from build123d import *

# Parameters (mm, degrees)
F0_W      = 70
F0_H      = 100
F1_DEPTH  = 19
F3_DEPTH  = 3
F4_R      = 16
F5_DEPTH  = 3
F7_DEPTH  = 3
F8_R      = 2
F9_DEPTH  = 3
F10_R     = 2
F11_DEPTH = 3


with BuildPart() as f1:
    # F0 (on Front) → F1 (new body)
    with BuildSketch(Plane.XZ):
        with Locations((35, -50)):
            Rectangle(F0_W, F0_H)
    extrude(amount=F1_DEPTH)

    # F2 (on face) → F3 (join)
    with BuildSketch(Plane.XZ.offset(19)):
        with BuildLine():
            Line((57, -8), (12, -8))
            Line((12, -8), (8, -11.356399))
            Line((8, -11.356399), (8, -86.344417))
            Line((8, -86.344417), (13.655583, -92))
            Line((13.655583, -92), (59, -92))
            ThreePointArc((59, -92), (61.162278, -90.576506), (62, -88.127017))
            Line((62, -88.127017), (62, -13))
            ThreePointArc((62, -13), (60.535534, -9.464466), (57, -8))
        make_face()
    extrude(amount=F3_DEPTH)

    # F4 (on face) → F5 (cut)
    with BuildSketch(Plane.XZ.offset(22)):
        with Locations((35, -30)):
            Circle(F4_R)
    extrude(amount=-F5_DEPTH, mode=Mode.SUBTRACT)

    # F6 (on face) → F7 (cut)
    with BuildSketch(Plane.XZ.offset(22)):
        with BuildLine():
            Line((47.590841, -64.431946), (29.590728, -64.431946))
            ThreePointArc((29.590728, -64.431946), (25.361132, -66.176302), (23.590841, -70.395109))
            Line((23.590841, -70.395109), (23.541725, -78.395109))
            ThreePointArc((23.541725, -78.395109), (25.285967, -82.661543), (29.541612, -84.431946))
            Line((29.541612, -84.431946), (47.590841, -84.431946))
            ThreePointArc((47.590841, -84.431946), (51.833482, -82.674587), (53.590841, -78.431946))
            Line((53.590841, -78.431946), (53.590841, -70.431946))
            ThreePointArc((53.590841, -70.431946), (51.833482, -66.189306), (47.590841, -64.431946))
        make_face()
    extrude(amount=-F7_DEPTH, mode=Mode.SUBTRACT)

    # F8 (on face) → F9 (cut)
    with BuildSketch(Plane.XZ.offset(22)):
        with Locations((10.5, -31.813467)):
            Circle(F8_R)
        with Locations((18.186533, -39.5)):
            Circle(F8_R)
        with BuildLine():
            ThreePointArc((19, -50), (21, -52), (23, -50))
            ThreePointArc((23, -50), (21, -48), (19, -50))
        make_face()
        with Locations((18.186533, -60.5)):
            Circle(F8_R)
        with Locations((10.5, -68.186533)):
            Circle(F8_R)
    extrude(amount=-F9_DEPTH, mode=Mode.SUBTRACT)

    # F10 (on face) → F11 (cut)
    with BuildSketch(Plane.XZ.offset(22)):
        with Locations((56, -40)):
            Circle(F10_R)
        with Locations((55.891707, -50)):
            Circle(F10_R)
        with Locations((56, -60)):
            Circle(F10_R)
    extrude(amount=-F11_DEPTH, mode=Mode.SUBTRACT)


solid = f1.part
Work out the finished part from the listing and answer in its coordinate system (mm). A direction names the side the tool comes from. Round coordinates to 2 decimals unless told otherwise and drop trailing zeros. Order: outer loops, then holes, each group sorted by start corner. A loop starts at its lowest first (then second) coordinate and runs counter-clockwise, first axis right, second up. Notation, with made-up numbers: M 27.25,26.25 L 60.25,26.25 A20 ccw 60.25,56.25 Z; hole C 15.5,-32.5 d11. An arc over 180 degrees is marked long. Put each result on its own line as item: value. Start each with the question number.
Q1. Section C-C, the plane y = -20 is taken. Give the number of separate pieces and of enclosed holes in the cut face, and give its area (3 significant figures).
Q2. Section D-D, the plane z = -75 is taken. Write down the section's boundary in (x, y).
Q3. For a pull along X with two mould halves and no side action, classify faces 1 (the flat face through (0, -9, -51)), 2 (the cylindrical face through (61.14, -20.479, -90.606)), 3 (the flat face through (3, -19, -49)), 4 (the flat face through (56, -19, -40)) as pulls with the +X half, pulls with the -X half, needs draft (parallel to the pull), parting line crosses it, or undercut.
Q4. A tool of negligible diameter and unlimited length cuts with its end or side. For faces 5 (the flat face through (10.028, -20.479, -9.655)), 6 (the flat face through (70, -9, -51)), 7 (the flat face through (8, -20, -48)), 8 (the cylindrical face through (51.79, -20.52, -82.72)), 9 (the flat face through (36, -20, -92)), from which of +Z, -Z, +X, -X, +Y, -Y can it reach the whole face along a straight path? Write none if from no direction.
Q5. Section A-A, the plane x = 35 is taken. Write down the section's boundary in (y, z), and give its area (3 significant figures).
Q6. Flat-ended cylindrical pins translate along their axes: pin 1 (5 mm diameter, centred on x = 24, y = -19.5, fed in from -Z); pin 2 (2 mm diameter, centred on x = 18, z = -39.5, fed in from -Y); pin 3 (3.5 mm diameter, centred on x = 43, y = -21, fed in from -Z); pin 4 (3.5 mm diameter, centred on y = -21, z = -37.5, fed in from +X). Find the tip coordinate at first contact, or state that the pin passes through.
Q7. Section B-B, the plane z = -50 is taken. Write down the section's boundary in (x, y).
Q8. Straight lines are drawn through the part: L1, parallel to Z at x = 35, y = -20.25; L2, parallel to Y at x = 25.5, z = -34; L3, parallel to X at y = -19.5, z = -55. For each, find the intervals that lie inside material, in ascending order. Write a range as [from, to].
Findings below:
1. separate pieces: 1
1. enclosed holes: 10
1. area: 3,030 mm^2
2. outline: M 0,-19 L 8,-19 L 8,-22 L 23.56,-22 L 23.56,-19 L 53.59,-19 L 53.59,-22 L 62,-22 L 62,-19 L 70,-19 L 70,0 L 0,0 Z
3. face 1: pulls with the -X half
3. face 2: pulls with the +X half
3. face 3: needs draft
3. face 4: undercut
4. face 5: +Z, -X, -Y
4. face 6: +Z, -Z, +X, +Y, -Y
4. face 7: +Z, -Z, -X, -Y
4. face 8: -Y
4. face 9: -Z, +X, -X, -Y
5. outline: M -22,-92 L -19,-92 L -19,-100 L 0,-100 L 0,0 L -19,0 L -19,-8 L -22,-8 L -22,-14 L -19,-14 L -19,-46 L -22,-46 L -22,-64.43 L -19,-64.43 L -19,-84.43 L -22,-84.43 Z
5. area: 2,000 mm^2
6. pin 1: stops at z = -100
6. pin 2: stops at y = -19
6. pin 3: stops at z = -92
6. pin 4: stops at x = 62
7. outline: M 0,-19 L 8,-19 L 8,-22 L 19,-22 L 19,-19 L 23,-19 L 23,-22 L 53.89,-22 L 53.89,-19 L 57.89,-19 L 57.89,-22 L 62,-22 L 62,-19 L 70,-19 L 70,0 L 0,0 Z
8. L1: z = [-92, -84.43], [-64.43, -46], [-14, -8]
8. L2: y = [-19, 0]
8. L3: x = [8, 62]
